```python
from build123d import *

# Parameters (mm, degrees)
BOSS_EXTRUDE1_DEPTH = 76.2
SKETCH2_W           = 64.3636
SKETCH2_H           = 77.0636
CUT_EXTRUDE1_DEPTH  = 400.05
SKETCH3_W           = 77.0636
SKETCH3_H           = 64.3636
CUT_EXTRUDE2_DEPTH  = 400.05
SWEEP2_START        = 19.05
SWEEP2_DEPTH        = 38.1
SKETCH12_R          = 7.9375
CUT_EXTRUDE3_DEPTH  = 400.05


# Read off the part's stored shape, not the designer's step: Sweep2
with BuildPart() as part:
    # Sketch1 → Boss-Extrude1 (new body)
    with BuildSketch(Plane.XY):
        Polygon((0, 0), (0, -317.5), (-88.9, -317.5), (-88.9, 88.9), (317.5, 88.9), (317.5, 0), align=None)
    extrude(amount=BOSS_EXTRUDE1_DEPTH)

    # Sketch2 → Cut-Extrude1 (cut)
    with BuildSketch(Plane(origin=(317.5, 0, 0), x_dir=(0, 0, -1), z_dir=(1, 0, 0))):
        with Locations((-38.1, 44.45)):
            Rectangle(SKETCH2_W, SKETCH2_H)
    extrude(amount=-CUT_EXTRUDE1_DEPTH, mode=Mode.SUBTRACT)

    # Sketch3 → Cut-Extrude2 (cut)
    with BuildSketch(Plane.XZ.offset(317.5)):
        with Locations((-44.45, 38.1)):
            Rectangle(SKETCH3_W, SKETCH3_H)
    extrude(amount=-CUT_EXTRUDE2_DEPTH, mode=Mode.SUBTRACT)

    # Sweep2 outline → Sweep2 (add)
    with BuildSketch(Plane.XY.offset(SWEEP2_START)):
        Polygon((0, -254.432954545), (0, -291.667045455), (298.45, 0), (260.35, 0), align=None)
    extrude(amount=SWEEP2_DEPTH)

    # Sketch12 → Cut-Extrude3 (cut)
    with BuildSketch(Plane(origin=(0, 0, 0), x_dir=(-1, 0, 0), z_dir=(0, 0, -1))):
        with Locations((44.45, -228.6)):
            Circle(SKETCH12_R)
        with Locations((44.45, -50.8)):
            Circle(SKETCH12_R)
        with Locations((-50.8, 44.45)):
            Circle(SKETCH12_R)
        with Locations((-228.6, 44.45)):
            Circle(SKETCH12_R)
    extrude(amount=-CUT_EXTRUDE3_DEPTH, mode=Mode.SUBTRACT)


solid = part.part
```
Input: part model. Units: mm. Frame: model coordinates. A direction names the side the tool comes from. Give positions to 0.01 mm unless a question says otherwise; leave off trailing zeros. Order: outer loops, then holes, each group sorted by start corner. A loop starts at its lowest first (then second) coordinate and runs counter-clockwise, first axis right, second up. Notation, with made-up numbers: (57, 76.25) - (61, 76.25) arc R23 cw to (61, 115.25) - close; hole circle Ø9 at (-36.5, -12). An arc over 180 degrees is marked (long way). One line per item, written item: value.
1. Cut plane C-C, the plane y = -68.5. Output: boundary loops of the cut face in (x, z), and give its area (3 significant figures).
Determined:
outline: (-88.9, 0) - (0, 0) - (0, 76.2) - (-88.9, 76.2) - close; (190.26, 19.05) - (228.36, 19.05) - (228.36, 57.15) - (190.26, 57.15) - close; hole (-82.98, 5.92) - (-5.92, 5.92) - (-5.92, 70.28) - (-82.98, 70.28) - close
area: 3,270 mm2
2. Cut plane B-B, the plane x = -44.45. Output: boundary loops of the cut face in (y, z), and give its area (3 significant figures).
Determined:
outline: (-317.5, 0) - (-236.54, 0) - (-236.54, 5.92) - (-317.5, 5.92) - close; (-317.5, 70.28) - (-236.54, 70.28) - (-236.54, 76.2) - (-317.5, 76.2) - close; (-220.66, 0) - (-58.74, 0) - (-58.74, 5.92) - (-220.66, 5.92) - close; (-220.66, 70.28) - (-58.74, 70.28) - (-58.74, 76.2) - (-220.66, 76.2) - close; (-42.86, 0) - (88.9, 0) - (88.9, 76.2) - (-42.86, 76.2) - (-42.86, 70.28) - (82.98, 70.28) - (82.98, 5.92) - (-42.86, 5.92) - close
area: 4,820 mm2
3. Draft query along Y for faces 5 (the face through (-38.15, -233.43, 73.2)), 6 (the face through (111, 88.9, 38)), 7 (the face through (317.5, 45, 71)), 8 (the face through (-44, -317.5, 71)). Return one class per face: released by +Y, released by -Y, zero draft, split by the parting line, or undercut.
Determined:
face 5: undercut
face 6: released by +Y
face 7: zero draft
face 8: released by -Y
4. Pin query (flat end, axial travel): pin 1 Ø12.5 at (x, y) = (50.8, 44.45) entering from -Z; pin 2 Ø0.5 at (y, z) = (82.5, 22.5) entering from +X; pin 3 Ø4 at (x, z) = (-45, 41.5) entering from -Y; pin 4 Ø0.5 at (x, z) = (-82.5, 23.5) entering from -Y. Return the tip coordinate at first contact, or that it passes through.
Determined:
pin 1: through
pin 2: x = -82.55
pin 3: y = 82.98
pin 4: y = 82.55
5. Line query: probe 1 along X at (y, z) = (44, 74); probe 2 along Y at (x, z) = (-44.45, 3.15); probe 3 along X at (y, z) = (-39.5, 66.5). Output: solid intervals per line, ascending.
Determined:
probe 1: -88.9 to 42.88, 58.72 to 220.68, 236.52 to 317.5
probe 2: -317.5 to -236.54, -220.66 to -58.74, -42.86 to 88.9
probe 3: -88.9 to -82.98, -5.92 to 0
6. Reachability of faces 1 (the face through (131.997, -125.435, 37.833)), 2 (the face through (158, 5.918, 39)), 3 (the face through (25, 13, 70.282)), 4 (the face through (-5.918, -158, 38)) from +Z, -Z, +X, -X, +Y, -Y: full face, straight path, thin tool, end or side. Return the list, or none.
Determined:
face 1: +Z, -Z
face 2: +X
face 3: none
face 4: -Y
7. Cut plane A-A, the plane z = 35.5. Output: boundary loops of the cut face in (x, y), and give its area (3 significant figures).
Determined:
outline: (-88.9, -317.5) - (-82.98, -317.5) - (-82.98, 82.55) - (-82.55, 82.55) - (-82.55, 82.98) - (317.5, 82.98) - (317.5, 88.9) - (-88.9, 88.9) - close; (-5.92, -317.5) - (0, -317.5) - (0, -291.67) - (298.45, 0) - (317.5, 0) - (317.5, 5.92) - (-5.92, 5.92) - close; hole (0, -254.43) - (260.35, 0) - (0, 0) - close
area: 19,000 mm2
8. Cut plane D-D, the plane x = 154. Output: boundary loops of the cut face in (y, z), and give its area (3 significant figures).
Determined:
outline: (-141.17, 19.05) - (-103.93, 19.05) - (-103.93, 57.15) - (-141.17, 57.15) - close; (0, 0) - (88.9, 0) - (88.9, 76.2) - (0, 76.2) - close; hole (5.92, 5.92) - (82.98, 5.92) - (82.98, 70.28) - (5.92, 70.28) - close
area: 3,230 mm2
